Here's how the part is built. I have some questions about the finished solid (model axes, mm). A direction names the side the tool comes from. Give positions to 0.01 mm unless a question says otherwise; leave off trailing zeros. Order: outer loops, then holes, each group sorted by start corner. A loop starts at its lowest first (then second) coordinate and runs counter-clockwise, first axis right, second up. Notation, with made-up numbers: (-15.75, 3.5) -> (32.25, 3.5) arc R22 cw to (32.25, 28.5) -> close; hole circle Ø7 at (-4.5, 10.25). An arc over 180 degrees is marked (long way). Write each question's results on one line, items separated by ' | '. Start each with the question number.
Q1. Thinking about a two-plate mould opening in Y: for faces 5 (the face through (-7.2, 29.5, 7.62)), 6 (the face through (-7.594, 29.377, 11.377)), 7 (the face through (-15.386, -45.135, 3.757)), 8 (the face through (-7.763, -37.025, 3.757)), which applies, pulls with the +Y half, pulls with the -Y half, needs draft (parallel to the pull), parting line crosses it, or undercut?
Q2. Imagine slicing it at A-A, the plane y = -34.5. Please give me the cut outline in (x, z).
Q3. Imagine slicing it at D-D, the plane x = -33.5. Please give me the cut outline in (y, z).
Q4. Imagine slicing it at C-C, the plane z = -4. Please give me the cut outline in (x, y).
Q5. I need wall thicknesses on line 1 along Z through (x, y) = (-12.5, -39); line 2 along Y through (x, z) = (-12.5, 4); line 3 along Y through (x, z) = (-18, 7.25). Which ranges of each line are inside material? Lowest first, please. Write a range as [from, to].
Q6. For faces 1 (the face through (-36.272, -24.352, 3.757)), 2 (the face through (-7.2, 29.5, 0)), 3 (the face through (-3.4, 20.1, -3.8)), 4 (the face through (-3.4, 20.1, 11.4)), which set-ups out of +Z, -Z, +X, -X, +Y, -Y let a thin tool reach every point of the face, with its end or its side?
Q7. Imagine slicing it at B-B, the plane z = 5.25. Please give me the cut outline in (x, y).
Q8. I'm going to push flat-ended pins straight in: pin 1 (1 mm diameter, centred on x = -0.5, y = -36.5, fed in from +Z); pin 2 (2 mm diameter, centred on x = -3.5, y = 12, fed in from -Z); pin 3 (3 mm diameter, centred on x = -14, z = -5, fed in from +Y); pin 4 (1 mm diameter, centred on x = -19, z = 8.5, fed in from +Y). Where does each tip first touch, or does it pass through?
```python
from build123d import *

# Parameters (mm, degrees)
F1_DEPTH      = 7.62
F3_DEPTH      = 7.62
F3_DEPTH_BACK = 15.24
F4_R          = 3.175
F5_DEPTH      = 79.502
F5_DEPTH_BACK = 34.798


with BuildPart() as f1:
    # F0 (on Top) → F1 (new body)
    with BuildSketch(Plane.XY):
        with BuildLine():
            ThreePointArc((-19.4344986555, 31.5148568491), (-1.0529688957, 9.7617744234), (5.5467668246, -17.9423898801))
            ThreePointArc((5.5467668246, -17.9423898801), (-8.0937566855, -37.1436695543), (-30.7152286304, -30.5845514882))
            Line((-30.7152286304, -30.5845514882), (-41.9875042541, -17.9423898801))
            ThreePointArc((-41.9875042541, -17.9423898801), (-14.7879740797, -45.1419200544), (12.4115560946, -17.9423898801))
            ThreePointArc((12.4115560946, -17.9423898801), (5.3194072823, 12.3671165466), (-14.4844366655, 36.3832053102))
            Line((-14.4844366655, 36.3832053102), (-19.4344986555, 31.5148568491))
        make_face()
    extrude(amount=F1_DEPTH)

    # F2 (on face) → F3 (join, two sides)
    with BuildSketch(Plane.XY.offset(7.62)) as f3_sk:
        with BuildLine():
            Line((-0.8935400487, 22.5641902395), (-14.4844366655, 36.3832053102))
            Line((-14.4844366655, 36.3832053102), (-19.4344986555, 31.5148568491))
            ThreePointArc((-19.4344986555, 31.5148568491), (-12.0907540568, 25.1445945609), (-5.8436020388, 17.6958417784))
            Line((-5.8436020388, 17.6958417784), (-0.8935400487, 22.5641902395))
        make_face()
    extrude(amount=F3_DEPTH)
    extrude(f3_sk.sketch, amount=-F3_DEPTH_BACK)

    # F4 (on face) → F5 (cut, two sides)
    with BuildSketch(Plane(origin=(10.8263263702, 10.6476099552, 0), x_dir=(-0.7011976155, 0.7129669726, 0), z_dir=(0.7129669726, 0.7011976155, 0))) as f5_sk:
        with Locations((26.4052733757, 3.81)):
            Circle(F4_R)
    extrude(amount=-F5_DEPTH, mode=Mode.SUBTRACT)
    extrude(f5_sk.sketch, amount=F5_DEPTH_BACK, mode=Mode.SUBTRACT)


solid = f1.part
```
Geometry check:
1) face 5: needs draft | face 6: pulls with the +Y half | face 7: pulls with the -Y half | face 8: undercut
2) outline: (-36.37, 0) -> (-26.59, 0) -> (-26.59, 7.62) -> (-36.37, 7.62) -> close; (-2.98, 0) -> (6.79, 0) -> (6.79, 7.62) -> (-2.98, 7.62) -> close
3) outline: (-37.68, 0) -> (-27.46, 0) -> (-27.46, 7.62) -> (-37.68, 7.62) -> close
4) outline: (-19.43, 31.51) arc R61.45 cw to (-5.84, 17.7) -> (-0.89, 22.56) -> (-14.48, 36.38) -> close
5) line 1: [0, 7.62] | line 2: [-45.05, -38.15], [29.19, 34.81] | line 3: [-44.95, -38.02], [30.42, 32.93]
6) face 1: +Z, -Z, +Y | face 2: -Z, +X, +Y | face 3: -Z, +X, -Y | face 4: +Z, +X, -Y
7) outline: (-41.99, -17.94) arc R27.2 ccw to (12.41, -17.94) arc R68.31 ccw to (-5.25, 27.9) -> (-10.15, 23.08) arc R61.45 cw to (5.55, -17.94) arc R20.33 cw to (-30.72, -30.58) -> close; (-19.43, 31.51) arc R61.45 cw to (-14.12, 27.12) -> (-9.22, 31.93) arc R68.31 ccw to (-14.48, 36.38) -> close
8) pin 1: z = 7.62 | pin 2: through | pin 3: y = 36.38 | pin 4: y = 32.43
